```python
from build123d import *

# Parameters (mm, degrees)
F0_R     = 25.4
F1_DEPTH = 25.4
F2_W     = 63.5
F2_H     = 63.5
F3_DEPTH = 25.4
F5_DEPTH = 63.501
F7_D     = 38.1
F7_DEPTH = 38.1
F7_TIP   = 11.4463947925


with BuildPart() as f1:
    # F0 (on Top) → F1 (new body)
    with BuildSketch(Plane.XY):
        Circle(F0_R)
    extrude(amount=F1_DEPTH)

    # F2 (on face) → F3 (join)
    with BuildSketch(Plane.XY):
        Rectangle(F2_W, F2_H)
    extrude(amount=-F3_DEPTH)

    # F4 (on face) → F5 (cut, through all)
    with BuildSketch(Plane.YZ.offset(31.75)):
        Polygon((-25.4, -19.05), (-16.51, -19.05), (-16.51, -25.4), (0, -25.4), (16.51, -25.4), (16.51, -19.05), (25.4, -19.05), (25.4, -15.05), (0, -15.05), (-25.4, -15.05), align=None)
    extrude(amount=-F5_DEPTH, mode=Mode.SUBTRACT)

    # F7
    with Locations(Plane.XY.offset(25.4)):
        with Locations((0, 0)):
            Hole(F7_D / 2, depth=F7_DEPTH)
            with Locations((0, 0, -(F7_DEPTH + F7_TIP / 2))):  # 118° drill point
                Cone(0, F7_D / 2, F7_TIP, mode=Mode.SUBTRACT)


solid = f1.part
```
Part model, mm, in its own coordinate system. A direction names the side the tool comes from. Coordinates: 2 decimals unless noted, no trailing zeros. Write each loop counter-clockwise with the first axis right and the second up, starting at its lowest first coordinate (ties: lowest second). Pieces come first, ordered by that corner, then holes.
Item 1: Slice it at B-B (x = 27). Write the cut outline in (y, z).
Item 2: Slice it at D-D (x = 0). Write the cut outline in (y, z).
Item 3: Slice it at A-A (z = -21). Write the cut outline in (x, y), and give its area (3 significant figures).
Item 4: Pin check, flat tips, straight feed: pin 1 (2 mm diameter, centred on x = -9.5, y = 13, fed in from -Z); pin 2 (6 mm diameter, centred on y = 10, z = 5.5, fed in from +X); pin 3 (1 mm diameter, centred on y = 3.5, z = 5, fed in from -X). Stop position of each tip, or through.
Item 5: Mould opens along Y. For faces 1 (the face through (0, -31.75, -13)), 2 (the face through (-22, 15, 0)), 3 (the face through (0, -21, -19.05)) say: released by +Y, released by -Y, zero draft, split by the parting line, or undercut.
Item 6: Slice it at C-C (y = 0). Write the cut outline in (x, z).
Item 7: Which spindle directions (+Z, -Z, +X, -X, +Y, -Y) get a long thin tool onto all of the face, cutting with end or side? Do faces 4 (the face through (0, 31.75, -13)), 5 (the face through (0, 21, -19.05)), 6 (the face through (0, -24, -25.4)), 7 (the face through (-5.506, -24.796, 12.522)), 8 (the face through (0, -16.51, -22)). Say none if no direction does.
Item 8: Probe line 1 (Y direction, x = 0, z = 9); line 2 (X direction, y = 0, z = -2); line 3 (Y direction, x = 9.5, z = -11). List the from-to ranges inside material, lowest first.
Results found:
1. outline: (-31.75, -25.4) - (-16.51, -25.4) - (-16.51, -19.05) - (-25.4, -19.05) - (-25.4, -15.05) - (25.4, -15.05) - (25.4, -19.05) - (16.51, -19.05) - (16.51, -25.4) - (31.75, -25.4) - (31.75, 0) - (-31.75, 0) - close
2. outline: (-31.75, -25.4) - (-16.51, -25.4) - (-16.51, -19.05) - (-25.4, -19.05) - (-25.4, -15.05) - (-15.14, -15.05) - (-19.05, -12.7) - (-19.05, 25.4) - (-25.4, 25.4) - (-25.4, 0) - (-31.75, 0) - close; (15.14, -15.05) - (25.4, -15.05) - (25.4, -19.05) - (16.51, -19.05) - (16.51, -25.4) - (31.75, -25.4) - (31.75, 0) - (25.4, 0) - (25.4, 25.4) - (19.05, 25.4) - (19.05, -12.7) - close
3. outline: (-31.75, -31.75) - (31.75, -31.75) - (31.75, -16.51) - (-31.75, -16.51) - close; (-31.75, 16.51) - (31.75, 16.51) - (31.75, 31.75) - (-31.75, 31.75) - close
3. area: 1,940 mm2
4. pin 1: stops at z = -15.05
4. pin 2: stops at x = 24.42
4. pin 3: stops at x = -25.22
5. face 1: released by -Y
5. face 2: zero draft
5. face 3: undercut
6. outline: (-31.75, -15.05) - (-15.14, -15.05) - (-19.05, -12.7) - (-19.05, 25.4) - (-25.4, 25.4) - (-25.4, 0) - (-31.75, 0) - close; (15.14, -15.05) - (31.75, -15.05) - (31.75, 0) - (25.4, 0) - (25.4, 25.4) - (19.05, 25.4) - (19.05, -12.7) - close
7. face 4: +Z, -Z, +X, -X, +Y
7. face 5: +X, -X
7. face 6: -Z, +X, -X, +Y, -Y
7. face 7: +Z
7. face 8: -Z, +X, -X
8. line 1: y = -25.4 to -19.05, 19.05 to 25.4
8. line 2: x = -31.75 to -19.05, 19.05 to 31.75
8. line 3: y = -31.75 to -16.51, 16.51 to 31.75
